from build123d import *

# Parameters (mm, degrees)
SKETCH1_W           = 94
SKETCH1_H           = 130
BOSS_EXTRUDE1_DEPTH = 5
SKETCH2_W           = 94
SKETCH2_H           = 130
SKETCH2_W_2         = 84
SKETCH2_H_2         = 120
BOSS_EXTRUDE2_DEPTH = 5
FILLET1_R           = 2
SKETCH3_W           = 44.1
SKETCH3_H           = 58.5
CUT_EXTRUDE1_DEPTH  = 2
SKETCH5_W           = 6
SKETCH5_H           = 6
BOSS_EXTRUDE4_DEPTH = 4
SKETCH7_R           = 1.20000014
CUT_EXTRUDE2_DEPTH  = 3
SKETCH8_W           = 54.6
SKETCH8_H           = 30
CUT_EXTRUDE3_DEPTH  = 3
SKETCH9_W           = 49.4
SKETCH9_H           = 27
CUT_EXTRUDE4_DEPTH  = 2
SKETCH10_W          = 49.4
SKETCH10_H          = 6.619549161
CUT_EXTRUDE5_DEPTH  = 2
SKETCH11_W          = 5
SKETCH11_H          = 1
CUT_EXTRUDE6_DEPTH  = 3
SKETCH14_W          = 84
SKETCH14_H          = 120
CUT_EXTRUDE8_DEPTH  = 2.5
SKETCH15_W          = 5
SKETCH15_H          = 5
BOSS_EXTRUDE5_DEPTH = 2.5
SKETCH16_R          = 1.5
CUT_EXTRUDE9_DEPTH  = 8.5
SKETCH17_R          = 2.8
CUT_EXTRUDE10_DEPTH = 3
SKETCH18_R          = 4
CUT_EXTRUDE11_DEPTH = 2


with BuildPart() as part:
    # Sketch1 → Boss-Extrude1 (new body)
    with BuildSketch(Plane(origin=(0, 0, 0), x_dir=(1, 0, 0), z_dir=(0, 1, 0))):
        with Locations((47, 65)):
            Rectangle(SKETCH1_W, SKETCH1_H)
    extrude(amount=BOSS_EXTRUDE1_DEPTH)

    # Sketch2 → Boss-Extrude2 (add)
    with BuildSketch(Plane(origin=(0, 5, 0), x_dir=(1, 0, 0), z_dir=(0, 1, 0))):
        with Locations((47, 65)):
            Rectangle(SKETCH2_W, SKETCH2_H)
        with Locations((47, 65)):
            Rectangle(SKETCH2_W_2, SKETCH2_H_2, mode=Mode.SUBTRACT)
    extrude(amount=BOSS_EXTRUDE2_DEPTH)

    # Fillet1
    fillet1_edges = [part.edges().sort_by_distance(p)[0] for p in [
        (47, 0, -130),
        (94, 0, -65),
        (47, 0, 0),
        (0, 0, -65),
        (0, 5, -130),
        (94, 5, -130),
        (94, 5, 0),
        (0, 5, 0),
    ]]
    fillet(fillet1_edges, radius=FILLET1_R)

    # Sketch3 → Cut-Extrude1 (cut)
    with BuildSketch(Plane(origin=(0, 5, 0), x_dir=(1, 0, 0), z_dir=(0, 1, 0))):
        with Locations((43.95, 44.25)):
            Rectangle(SKETCH3_W, SKETCH3_H)
    extrude(amount=-CUT_EXTRUDE1_DEPTH, mode=Mode.SUBTRACT)

    # Sketch5 → Boss-Extrude4 (add)
    with BuildSketch(Plane(origin=(0, 3, 0), x_dir=(1, 0, 0), z_dir=(0, 1, 0))):
        with Locations((24.9, 70.5)):
            Rectangle(SKETCH5_W, SKETCH5_H)
        with Locations((63, 70.5)):
            Rectangle(SKETCH5_W, SKETCH5_H)
        with Locations((63, 18)):
            Rectangle(SKETCH5_W, SKETCH5_H)
        with Locations((24.9, 18)):
            Rectangle(SKETCH5_W, SKETCH5_H)
    extrude(amount=BOSS_EXTRUDE4_DEPTH)

    # Sketch7 → Cut-Extrude2 (cut)
    with BuildSketch(Plane(origin=(0, 7, 0), x_dir=(1, 0, 0), z_dir=(0, 1, 0))):
        with Locations((25.710000549, 69.839000092)):
            Circle(SKETCH7_R)
        with Locations((62.514600549, 69.839000092)):
            Circle(SKETCH7_R)
        with Locations((62.514600549, 18.835800092)):
            Circle(SKETCH7_R)
        with Locations((25.710000549, 18.835800092)):
            Circle(SKETCH7_R)
    extrude(amount=-CUT_EXTRUDE2_DEPTH, mode=Mode.SUBTRACT)

    # Sketch8 → Cut-Extrude3 (cut)
    with BuildSketch(Plane(origin=(0, 5, 0), x_dir=(1, 0, 0), z_dir=(0, 1, 0))):
        with Locations((47, 110)):
            Rectangle(SKETCH8_W, SKETCH8_H)
    extrude(amount=-CUT_EXTRUDE3_DEPTH, mode=Mode.SUBTRACT)

    # Sketch9 → Cut-Extrude4 (cut)
    with BuildSketch(Plane(origin=(0, 2, 0), x_dir=(1, 0, 0), z_dir=(0, 1, 0))):
        with Locations((47, 110)):
            Rectangle(SKETCH9_W, SKETCH9_H)
    extrude(amount=-CUT_EXTRUDE4_DEPTH, mode=Mode.SUBTRACT)

    # Sketch10 → Cut-Extrude5 (cut)
    with BuildSketch(Plane.XZ):
        with Locations((47, -126.809774581)):
            Rectangle(SKETCH10_W, SKETCH10_H)
    extrude(amount=-CUT_EXTRUDE5_DEPTH, mode=Mode.SUBTRACT)

    # Sketch11 → Cut-Extrude6 (cut)
    with BuildSketch(Plane(origin=(0, 0, -96.5), x_dir=(-1, 0, 0), z_dir=(0, 0, -1))):
        with Locations((-47, 1)):
            Rectangle(SKETCH11_W, SKETCH11_H)
    extrude(amount=-CUT_EXTRUDE6_DEPTH, mode=Mode.SUBTRACT)

    # Sketch14 → Cut-Extrude8 (cut)
    with BuildSketch(Plane(origin=(0, 10, 0), x_dir=(1, 0, 0), z_dir=(0, 1, 0))):
        with BuildLine():
            Line((92.5, 2), (92.5, 128))
            ThreePointArc((92.5, 128), (92.353553391, 128.353553391), (92, 128.5))
            Line((92, 128.5), (2, 128.5))
            ThreePointArc((2, 128.5), (1.646446609, 128.353553391), (1.5, 128))
            Line((1.5, 128), (1.5, 2))
            ThreePointArc((1.5, 2), (1.646446609, 1.646446609), (2, 1.5))
            Line((2, 1.5), (92, 1.5))
            ThreePointArc((92, 1.5), (92.353553391, 1.646446609), (92.5, 2))
        make_face()
        with Locations((47, 65)):
            Rectangle(SKETCH14_W, SKETCH14_H, mode=Mode.SUBTRACT)
    extrude(amount=-CUT_EXTRUDE8_DEPTH, mode=Mode.SUBTRACT)

    # Sketch15 → Boss-Extrude5 (add)
    with BuildSketch(Plane(origin=(0, 5, 0), x_dir=(1, 0, 0), z_dir=(0, 1, 0))):
        with Locations((86.5, 122.5)):
            Rectangle(SKETCH15_W, SKETCH15_H)
        with Locations((7.5, 122.5)):
            Rectangle(SKETCH15_W, SKETCH15_H)
        with Locations((7.5, 7.5)):
            Rectangle(SKETCH15_W, SKETCH15_H)
        with Locations((86.5, 7.5)):
            Rectangle(SKETCH15_W, SKETCH15_H)
    extrude(amount=BOSS_EXTRUDE5_DEPTH)

    # Sketch16 → Cut-Extrude9 (cut, through all)
    with BuildSketch(Plane(origin=(0, 7.5, 0), x_dir=(1, 0, 0), z_dir=(0, 1, 0))):
        with Locations((6.5, 123.5)):
            Circle(SKETCH16_R)
        with Locations((87.5, 123.5)):
            Circle(SKETCH16_R)
        with Locations((87.5, 6.5)):
            Circle(SKETCH16_R)
        with Locations((6.5, 6.5)):
            Circle(SKETCH16_R)
    extrude(amount=-CUT_EXTRUDE9_DEPTH, mode=Mode.SUBTRACT)

    # Sketch17 → Cut-Extrude10 (cut)
    with BuildSketch(Plane.XZ):
        with Locations((6.5, -6.5)):
            Circle(SKETCH17_R)
        with Locations((87.5, -6.5)):
            Circle(SKETCH17_R)
        with Locations((87.5, -123.5)):
            Circle(SKETCH17_R)
        with Locations((6.5, -123.5)):
            Circle(SKETCH17_R)
    extrude(amount=-CUT_EXTRUDE10_DEPTH, mode=Mode.SUBTRACT)

    # Sketch18 → Cut-Extrude11 (cut)
    with BuildSketch(Plane.XZ):
        with Locations((6.5, -123.5)):
            Circle(SKETCH18_R)
        with Locations((87.5, -123.5)):
            Circle(SKETCH18_R)
        with Locations((87.5, -6.5)):
            Circle(SKETCH18_R)
        with Locations((6.5, -6.5)):
            Circle(SKETCH18_R)
    extrude(amount=-CUT_EXTRUDE11_DEPTH, mode=Mode.SUBTRACT)


solid = part.part
For this review, take the finished solid that the model builds, in its own axes (mm). A direction names the side the tool comes from. Round coordinates to 2 decimals unless told otherwise and drop trailing zeros. Order: outer loops, then holes, each group sorted by start corner. A loop starts at its lowest first (then second) coordinate and runs counter-clockwise, first axis right, second up. Notation, with made-up numbers: M -1.75,31 L 31.25,31 A21 ccw 31.25,51 Z; hole C 19,11.5 d4. An arc over 180 degrees is marked long. Use a Markdown table: item, result. Add a question column.
Item 1: Add section D-D, the plane z = -6.5. State how many separate pieces and enclosed holes the cut face has, then the cut area to 3 significant figures.
Item 2: Tool access review of faces 4 (the flat face through (47, 1.5, -95)), 5 (the flat face through (8, 3, -125)), 6 (the flat face through (3, 7.5, -65)): name each direction out of +Z, -Z, +X, -X, +Y, -Y from which nothing blocks a thin tool from reaching the whole face with its end or side.
Item 3: Add section A-A, the plane x = 55. Give the boundary of the cut face in (y, z), then the cut area to 3 significant figures.
Item 4: To check wall thickness, follow line 1 along X through (y, z) = (6.25, -123.5); line 2 along Z through (x, y) = (87.5, 2.5); line 3 along Z through (x, y) = (87.5, 5.05). State the ranges of each line that lie inside material, in increasing order.
Item 5: Add section C-C, the plane x = 77.5. Give the boundary of the cut face in (y, z), then the cut area to 3 significant figures.
Item 6: Add section B-B, the plane z = -25. Give the boundary of the cut face in (x, y), then the cut area to 3 significant figures.
Item 7: Mouldability with a two-part tool opening along X and no side actions: class faces 1 (the cylindrical face through (83.504, 0.986, -6.324)), 2 (the flat face through (0, 6, -64)), 3 (the flat face through (46, 0, -52)) as released by +X, released by -X, zero draft, split by the parting line, or undercut.
Item 8: Insertion check: pin 1 (6.5 mm diameter, centred on x = 6.5, z = -123.5, fed in from +Y); pin 2 (1.4 mm diameter, centred on x = 25.71, z = -18.84, fed in from +Y); pin 3 (4 mm diameter, centred on x = 63.5, z = -53, fed in from -Y); pin 4 (6.5 mm diameter, centred on x = 23.5, z = -70.5, fed in from +Y). Each pin has a flat end and moves straight along its axis. Give the tip position at first contact, or say it passes through.
Geometry results:
| question | item | result |
|---|---|---|
| 1 | separate pieces | 3 |
| 1 | enclosed holes | 0 |
| 1 | area | 456 mm² |
| 2 | face 4 | -Z |
| 2 | face 5 | -Y |
| 2 | face 6 | +Y |
| 3 | outline | M 0,-96.5 L 2,-96.5 L 2,-95 L 5,-95 L 5,-73.5 L 3,-73.5 L 3,-15 L 5,-15 L 5,-5 L 7.5,-5 L 7.5,-1.5 L 10,-1.5 L 10,0 L 2,0 A2 ccw 0,-2 Z; M 2,-130 L 10,-130 L 10,-128.5 L 7.5,-128.5 L 7.5,-125 L 2,-125 Z |
| 3 | area | 408 mm² |
| 4 | line 1 | x = 0 to 5, 8 to 10, 84 to 86, 89 to 94 |
| 4 | line 2 | z = -130 to -126.3, -120.7 to -9.3, -3.7 to 0 |
| 4 | line 3 | z = -130 to -125, -122 to -120, -10 to -8, -5 to 0 |
| 5 | outline | M 0,-128 A2 ccw 2,-130 L 10,-130 L 10,-128.5 L 7.5,-128.5 L 7.5,-125 L 5,-125 L 5,-5 L 7.5,-5 L 7.5,-1.5 L 10,-1.5 L 10,0 L 2,0 A2 ccw 0,-2 Z |
| 5 | area | 681 mm² |
| 6 | outline | M 0,2 A2 ccw 2,0 L 92,0 A2 ccw 94,2 L 94,10 L 92.5,10 L 92.5,7.5 L 89,7.5 L 89,5 L 66,5 L 66,3 L 21.9,3 L 21.9,5 L 5,5 L 5,7.5 L 1.5,7.5 L 1.5,10 L 0,10 Z |
| 6 | area | 413 mm² |
| 7 | face 1 | undercut |
| 7 | face 2 | released by -X |
| 7 | face 3 | zero draft |
| 8 | pin 1 | stops at y = 7.5 |
| 8 | pin 2 | stops at y = 4 |
| 8 | pin 3 | stops at y = 0 |
| 8 | pin 4 | stops at y = 7 |
